Geometry check sheet. Reference: the model listing, model coordinates, mm. Face numbers are marked on the shaded views. A direction names the side the tool comes from. Give positions to 0.01 mm unless a question says otherwise; leave off trailing zeros. Loops run counter-clockwise (first coordinate to the right, second up) from the corner with the lowest first, then second, coordinate; pieces in that order, holes last. Notation, with made-up numbers: (76, -34) - (132, -34) arc R30 ccw to (132, -3) - close; hole circle Ø8 at (64, 76). An arc over 180 degrees is marked (long way). Use a Markdown table: item, result. Add a question column.
1. Cross-section at C-C on y = -5.08. Enter the section's corners in (x, z).
2. Depth check by flat-ended pin: P1, Ø10, axis at x = 18, y = -17.5, coming from the -Z side; P2, Ø7, axis at x = -14.5, z = 4.5, coming from the -Y side. Enter the tip coordinate at first touch or a pass-through.
3. Set-up check for the marked faces 1 and 2: record each of +Z, -Z, +X, -X, +Y, -Y from which the full face is reachable in a straight line by a thin tool's end or side.
4. Material ranges on L1, parallel to X at y = -6, z = 16; L2, parallel to Y at x = 40, z = 9.25; L3, parallel to X at y = -5.5, z = 7.5, recorded low to high.
5. Cross-section at D-D on x = 58.5. Enter the section's corners in (y, z), and give its area (3 significant figures).
6. Cross-section at B-B on y = -16.5. Enter the section's corners in (x, z), and give its area (3 significant figures).
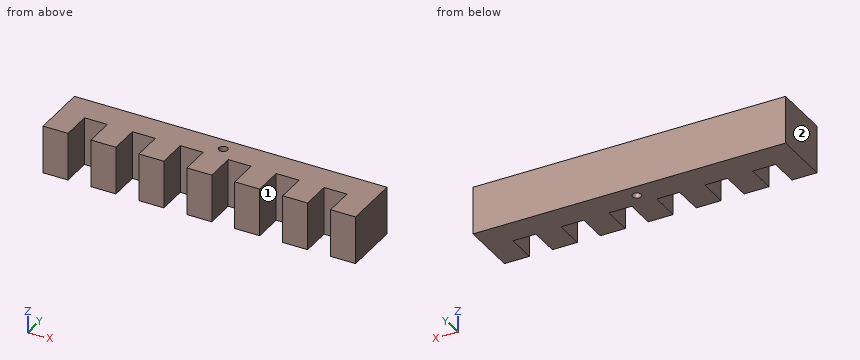
from build123d import *

# Parameters (mm, degrees)
F0_R     = 1.651
F1_DEPTH = 18.034


with BuildPart() as f1:
    # F0 (on Top) → F1 (new body)
    with BuildSketch(Plane.XY):
        Polygon((70.612, 0), (-46.99, 0), (-46.99, -21.336), (-37.592, -21.336), (-37.592, -10.16), (-28.956, -10.16), (-28.956, -21.336), (-19.558, -21.336), (-19.558, -10.16), (-10.922, -10.16), (-10.922, -21.336), (-1.524, -21.336), (-1.524, -10.16), (7.112, -10.16), (7.112, -21.336), (16.51, -21.336), (16.51, -10.16), (25.146, -10.16), (25.146, -21.336), (34.544, -21.336), (34.544, -10.16), (43.18, -10.16), (43.18, -21.336), (52.578, -21.336), (52.578, -10.16), (61.214, -10.16), (61.214, -21.336), (70.612, -21.336), align=None)
        with Locations((11.810999, -5.08)):
            Circle(F0_R, mode=Mode.SUBTRACT)
    extrude(amount=F1_DEPTH)


solid = f1.part
Values found:
| question | item | result |
|---|---|---|
| 1 | outline | (-46.99, 0) - (10.16, 0) - (10.16, 18.03) - (-46.99, 18.03) - close; (13.46, 0) - (70.61, 0) - (70.61, 18.03) - (13.46, 18.03) - close |
| 2 | P1 | stops at z = 0 |
| 2 | P2 | stops at y = -10.16 |
| 3 | face 1 | +Z, -Z, -Y |
| 3 | face 2 | +Z, -Z, -X, +Y, -Y |
| 4 | L1 | x = -46.99 to 10.44, 13.18 to 70.61 |
| 4 | L2 | y = -10.16 to 0 |
| 4 | L3 | x = -46.99 to 10.21, 13.41 to 70.61 |
| 5 | outline | (-10.16, 0) - (0, 0) - (0, 18.03) - (-10.16, 18.03) - close |
| 5 | area | 183 mm2 |
| 6 | outline | (-46.99, 0) - (-37.59, 0) - (-37.59, 18.03) - (-46.99, 18.03) - close; (-28.96, 0) - (-19.56, 0) - (-19.56, 18.03) - (-28.96, 18.03) - close; (-10.92, 0) - (-1.52, 0) - (-1.52, 18.03) - (-10.92, 18.03) - close; (7.11, 0) - (16.51, 0) - (16.51, 18.03) - (7.11, 18.03) - close; (25.15, 0) - (34.54, 0) - (34.54, 18.03) - (25.15, 18.03) - close; (43.18, 0) - (52.58, 0) - (52.58, 18.03) - (43.18, 18.03) - close; (61.21, 0) - (70.61, 0) - (70.61, 18.03) - (61.21, 18.03) - close |
| 6 | area | 1,190 mm2 |
